Model file for the job. Use its own axes, mm. Face numbers are marked on the shaded views. A direction names the side the tool comes from. Round coordinates to 2 decimals unless told otherwise and drop trailing zeros. Loops run counter-clockwise (first coordinate to the right, second up) from the corner with the lowest first, then second, coordinate; pieces in that order, holes last. Notation, with made-up numbers: (85, 89.5) - (112, 89.5) arc R30 ccw to (112, 128.5) - close; hole circle Ø3 at (-19.5, 18). An arc over 180 degrees is marked (long way). Answer as a JSON object with one key per item and string values.
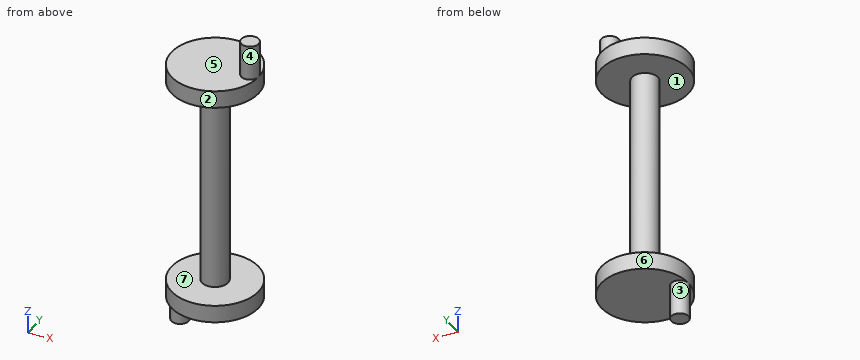
from build123d import *

# Parameters (mm, degrees)
SKETCH1_R           = 2.5
BOSS_EXTRUDE1_DEPTH = 1
SKETCH1_3_R         = 0.75
BOSS_EXTRUDE2_DEPTH = 12
BOSS_EXTRUDE4_START = 1
SKETCH1_5_R         = 0.5
BOSS_EXTRUDE4_DEPTH = 2
BOSS_EXTRUDE6_START = -13
SKETCH1_7_R         = 2.5
BOSS_EXTRUDE6_DEPTH = 1
BOSS_EXTRUDE7_START = -13
SKETCH1_8_R         = 0.5
BOSS_EXTRUDE7_DEPTH = 2


with BuildPart() as part:
    # Sketch1 → Boss-Extrude1 (new body)
    with BuildSketch(Plane.XY):
        Circle(SKETCH1_R)
    extrude(amount=BOSS_EXTRUDE1_DEPTH)

    # Sketch1<3> → Boss-Extrude2 (add)
    with BuildSketch(Plane.XY):
        Circle(SKETCH1_3_R)
    extrude(amount=-BOSS_EXTRUDE2_DEPTH)

    # Sketch1<5> → Boss-Extrude4 (add)
    with BuildSketch(Plane.XY.offset(BOSS_EXTRUDE4_START)):
        with Locations((2, 0)):
            Circle(SKETCH1_5_R)
    extrude(amount=BOSS_EXTRUDE4_DEPTH)

    # Sketch1<7> → Boss-Extrude6 (add)
    with BuildSketch(Plane.XY.offset(BOSS_EXTRUDE6_START)):
        Circle(SKETCH1_7_R)
    extrude(amount=BOSS_EXTRUDE6_DEPTH)

    # Sketch1<8> → Boss-Extrude7 (add)
    with BuildSketch(Plane.XY.offset(BOSS_EXTRUDE7_START)):
        with Locations((-2, 0)):
            Circle(SKETCH1_8_R)
    extrude(amount=-BOSS_EXTRUDE7_DEPTH)


solid = part.part
1) Tool access for the marked faces 1, 2, 3 and 4: list every direction of +Z, -Z, +X, -X, +Y, -Y with a clear straight run to the whole face (end or side of a thin tool).
Values follow:
{"face 1": "none", "face 2": "+Z, -Z", "face 3": "-Z", "face 4": "+Z"}
2) Slice it at C-C on x = 0.5. List the corners of the cut face in (y, z), then the cut area to 3 significant figures.
Values follow:
{"outline": "(-2.45, -13) - (2.45, -13) - (2.45, -12) - (0.56, -12) - (0.56, 0) - (2.45, 0) - (2.45, 1) - (-2.45, 1) - (-2.45, 0) - (-0.56, 0) - (-0.56, -12) - (-2.45, -12) - close", "area": "23.2 mm²"}
3) Drop flat-ended pins along their axis: P1, Ø2.5, axis at x = -0.5, y = -0.5, coming from the -Z side; P2, Ø1.5, axis at x = 1, y = -1, coming from the -Z side; P3, Ø2.5, axis at x = 0, y = -0.5, coming from the +Z side; P4, Ø1, axis at x = 0, z = -4, coming from the -Y side. Give the stop position or say it passes through.
Values follow:
{"P1": "z = -15", "P2": "z = -13", "P3": "z = 1", "P4": "y = -0.75"}
4) Slice it at A-A on x = 2. List the corners of the cut face in (y, z).
Values follow:
{"outline": "(-1.5, -13) - (1.5, -13) - (1.5, -12) - (-1.5, -12) - close; (-1.5, 0) - (1.5, 0) - (1.5, 1) - (0.5, 1) - (0.5, 3) - (-0.5, 3) - (-0.5, 1) - (-1.5, 1) - close"}
5) Two-plate mould, pull along Z, no slides. Class the marked faces 5, 6 and 7: pulls with the +Z half, pulls with the -Z half, needs draft (parallel to the pull), parting line crosses it, or undercut.
Values follow:
{"face 5": "pulls with the +Z half", "face 6": "needs draft", "face 7": "undercut"}
6) Slice it at B-B on y = -1.15. List the corners of the cut face in (x, z), then the cut area to 3 significant figures.
Values follow:
{"outline": "(-2.22, -13) - (2.22, -13) - (2.22, -12) - (-2.22, -12) - close; (-2.22, 0) - (2.22, 0) - (2.22, 1) - (-2.22, 1) - close", "area": "8.88 mm²"}
7) Probe probe 1 along Z at (x, y) = (0, 1.9); probe 2 along Y at (x, z) = (0, -3.25); probe 3 along Y at (x, z) = (1.95, 1.75). List the from-to ranges inside material, lowest first.
Values follow:
{"probe 1": "-13 to -12, 0 to 1", "probe 2": "-0.75 to 0.75", "probe 3": "-0.5 to 0.5"}
8) Slice it at D-D on z = -12.5. List the corners of the cut face in (x, y).
Values follow:
{"outline": "circle Ø5 at (0, 0)"}
